from build123d import *

# Parameters (mm, degrees)
F0_R     = 15.875
F3_DEPTH = 3.175
F1_R     = 12.7
F4_DEPTH = 25.4
F2_R     = 9.525
F5_DEPTH = 25.4


with BuildPart() as f3:
    # F0 (on Front) → F3 (new body)
    with BuildSketch(Plane.XZ):
        Circle(F0_R)
    extrude(amount=F3_DEPTH)

    # F1 (on Front) → F4 (join)
    with BuildSketch(Plane.XZ):
        Circle(F1_R)
    extrude(amount=F4_DEPTH)

    # F2 (on Front) → F5 (cut)
    with BuildSketch(Plane.XZ):
        Circle(F2_R)
    extrude(amount=F5_DEPTH, mode=Mode.SUBTRACT)


solid = f3.part
Can you work these out from the model? Positions are in its coordinate system, mm. A direction names the side the tool comes from. Round coordinates to 2 decimals unless told otherwise and drop trailing zeros. Order: outer loops, then holes, each group sorted by start corner. A loop starts at its lowest first (then second) coordinate and runs counter-clockwise, first axis right, second up. Notation, with made-up numbers: (50, 71) -> (55, 71) arc R14 cw to (55, 83) -> close; hole circle Ø10 at (-9.75, 1.25). An arc over 180 degrees is marked (long way). Write each question's results on one line, items separated by ' | '. Start each with the question number.
Item 1: Please list where these lines run through material, in increasing order: L1, parallel to Z at x = 0, y = -11 (3 decimals); L2, parallel to Y at x = 0, z = -13 (3 decimals); L3, parallel to Z at x = 7, y = -9.
Item 2: Will these pins go through, and if not, where does the flat tip stop? pin 1 (2 mm diameter, centred on x = -5, y = -8, fed in from -Z); pin 2 (6 mm diameter, centred on x = 6.5, y = -6, fed in from -Z); pin 3 (3 mm diameter, centred on y = -6, z = -11.5, fed in from -X); pin 4 (3 mm diameter, centred on x = -5.5, z = 7, fed in from +Y).
Item 3: If we section it at A-A, the plane z = 0: Write out the boundary of the cut face in (x, y) (3 decimals), then the cut area to 3 significant figures.
Item 4: Thinking about a two-plate mould opening in Z: for faces 1 (the cylindrical face through (-3.441, -1.565, -15.497)), 2 (the flat face through (-7, -3.175, 11)), 3 (the cylindrical face through (-7.559, -12.522, -5.796)), which applies, +Z half, -Z half, draft (parallel to the pull), parting line (faces both ways), or undercut?
Item 5: Which directions (+Z, -Z, +X, -X, +Y, -Y) give clear straight access to the entire face, cutting with the end or side of a thin tool? Please do faces 4 (the flat face through (5, -25.4, 9)), 5 (the cylindrical face through (-2.75, -14.13, -12.4)).
Item 6: If we section it at D-D, the plane x = -11: Write out the boundary of the cut face in (y, z) (3 decimals), then the cut area to 3 significant figures.
Item 7: If we section it at B-B, the plane x = 0: Write out the boundary of the cut face in (y, z) (3 decimals), then the cut area to 3 significant figures.
Item 8: If we section it at C-C, the plane y = -10: Write out the boundary of the cut face in (x, z) (3 decimals), then the cut area to 3 significant figures.
Results:
1) L1: z = -12.7 to -9.525, 9.525 to 12.7 | L2: y = -3.175 to 0 | L3: z = -10.6 to -6.46, 6.46 to 10.6
2) pin 1: stops at z = -12.05 | pin 2: stops at z = -14.9 | pin 3: stops at x = -7.83 | pin 4: stops at y = 0
3) outline: (-15.875, -3.175) -> (-12.7, -3.175) -> (-12.7, -25.4) -> (-9.525, -25.4) -> (-9.525, 0) -> (-15.875, 0) -> close; (9.525, -25.4) -> (12.7, -25.4) -> (12.7, -3.175) -> (15.875, -3.175) -> (15.875, 0) -> (9.525, 0) -> close | area: 181 mm2
4) face 1: parting line | face 2: draft | face 3: undercut
5) face 4: +Z, -Z, +X, -X, -Y | face 5: -Y
6) outline: (-25.4, -6.347) -> (-3.175, -6.347) -> (-3.175, -11.446) -> (0, -11.446) -> (0, 11.446) -> (-3.175, 11.446) -> (-3.175, 6.347) -> (-25.4, 6.347) -> close | area: 355 mm2
7) outline: (-25.4, -12.7) -> (-3.175, -12.7) -> (-3.175, -15.875) -> (0, -15.875) -> (0, -9.525) -> (-25.4, -9.525) -> close; (-25.4, 9.525) -> (0, 9.525) -> (0, 15.875) -> (-3.175, 15.875) -> (-3.175, 12.7) -> (-25.4, 12.7) -> close | area: 181 mm2
8) outline: circle Ø25.4 at (0, 0); hole circle Ø19.05 at (0, 0) | area: 222 mm2
